```python
from build123d import *

# Parameters (mm, degrees)
BOSS_EXTRUDE1_DEPTH = 10.16
SKETCH2_R           = 6.35
CUT_EXTRUDE1_DEPTH  = 25.4
CHAMFER1_SIZE       = 2.54
CHAMFER2_SIZE       = 2.54


with BuildPart() as part:
    # Sketch1 → Boss-Extrude1 (new body)
    with BuildSketch(Plane.XY):
        Polygon((-34.042504308, -19.37463512), (16.757495692, -19.37463512), (16.757495692, 12.37536488), (10.407495692, 12.37536488), (10.407495692, -13.02463512), (-27.692504308, -13.02463512), (-27.692504308, 12.37536488), (-34.042504308, 12.37536488), align=None)
    extrude(amount=BOSS_EXTRUDE1_DEPTH)

    # Sketch2 → Cut-Extrude1 (cut)
    with BuildSketch(Plane.XY.offset(10.16)):
        with Locations((-38.614504308, 3.48536488)):
            Circle(SKETCH2_R)
        with Locations((21.329495692, 3.48536488)):
            Circle(SKETCH2_R)
    extrude(amount=-CUT_EXTRUDE1_DEPTH, mode=Mode.SUBTRACT)

    # Chamfer1
    chamfer1_edges = [part.edges().sort_by_distance(p)[0] for p in [
        (16.757495692, 12.37536488, 5.08),
    ]]
    chamfer(chamfer1_edges, length=CHAMFER1_SIZE)

    # Chamfer2
    chamfer2_edges = [part.edges().sort_by_distance(p)[0] for p in [
        (-34.042504308, 12.37536488, 5.08),
    ]]
    chamfer(chamfer2_edges, length=CHAMFER2_SIZE)


solid = part.part
```
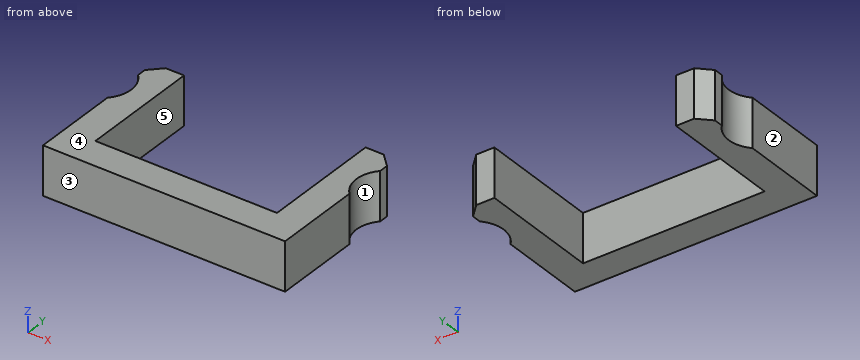
Part model, mm, in its own coordinate system. Face numbers are marked on the shaded views. A direction names the side the tool comes from. Round coordinates to 2 decimals unless told otherwise and drop trailing zeros. Write each loop counter-clockwise with the first axis right and the second up, starting at its lowest first coordinate (ties: lowest second). Pieces come first, ordered by that corner, then holes.
Item 1: Which spindle directions (+Z, -Z, +X, -X, +Y, -Y) get a long thin tool onto all of the face, cutting with end or side? Do the marked faces 4 and 5. Say none if no direction does.
Results:
face 4: +Z, +X, -X, +Y, -Y
face 5: +Z, -Z, +Y
Item 2: Cut at B-B, the plane z = 3. Give the cut face in (x, y), plus the area to 3 significant figures.
Results:
outline: (-34.04, -19.37) - (16.76, -19.37) - (16.76, -0.92) arc R6.35 cw to (16.76, 7.89) - (16.76, 9.84) - (14.22, 12.38) - (10.41, 12.38) - (10.41, -13.02) - (-27.69, -13.02) - (-27.69, 12.38) - (-31.5, 12.38) - (-34.04, 9.84) - (-34.04, 7.89) arc R6.35 cw to (-34.04, -0.92) - close
area: 617 mm2
Item 3: Cut at D-D, the plane y = 7. Give the cut face in (x, z).
Results:
outline: (-33.33, 0) - (-27.69, 0) - (-27.69, 10.16) - (-33.33, 10.16) - close; (10.41, 0) - (16.04, 0) - (16.04, 10.16) - (10.41, 10.16) - close
Item 4: Two-plate mould, pull along Y, no slides. Class the marked faces 1, 2 and 3: +Y half, -Y half, draft (parallel to the pull), parting line (faces both ways), or undercut.
Results:
face 1: undercut
face 2: draft
face 3: -Y half
Item 5: Probe L1, parallel to X at y = -8, z = 8.5; L2, parallel to X at y = 3.5, z = 4.5; L3, parallel to Y at x = 2.5, z = 6. List the from-to ranges inside material, lowest first.
Results:
L1: x = -34.04 to -27.69, 10.41 to 16.76
L2: x = -32.26 to -27.69, 10.41 to 14.98
L3: y = -19.37 to -13.02
Item 6: Cut at C-C, the plane x = -21. Give the cut face in (y, z), plus the area to 3 significant figures.
Results:
outline: (-19.37, 0) - (-13.02, 0) - (-13.02, 10.16) - (-19.37, 10.16) - close
area: 64.5 mm2
Item 7: Cut at A-A, the plane y = -2.5. Give the cut face in (x, z), plus the area to 3 significant figures.
Results:
outline: (-34.04, 0) - (-27.69, 0) - (-27.69, 10.16) - (-34.04, 10.16) - close; (10.41, 0) - (16.76, 0) - (16.76, 10.16) - (10.41, 10.16) - close
area: 129 mm2
Item 8: Drop a flat-ended pin along its axis: pin 1 Ø3 at (y, z) = (4.5, 3.5) entering from -X. Give the stop position or say it passes through.
Results:
pin 1: stops at x = -32.78
